from build123d import *

# Parameters (mm, degrees)
SKETCH1_W           = 1500
SKETCH1_H           = 1250
BOSS_EXTRUDE1_DEPTH = 150
CUT_EXTRUDE1_REACH  = 1633.908
LPATTERN1_COUNT     = 4
LPATTERN1_PITCH     = 150
LPATTERN1_COL_COUNT = 4
LPATTERN1_COL_PITCH = 150
CUT_EXTRUDE2_REACH  = 1467.435
SKETCH3_W           = 22
SKETCH3_H           = 11
LPATTERN2_COUNT     = 2
LPATTERN2_PITCH     = 525
LPATTERN2_COL_COUNT = 2
LPATTERN2_COL_PITCH = 525
CHAMFER1_SIZE       = 125


with BuildPart() as part:
    # Sketch1 → Boss-Extrude1 (new body)
    with BuildSketch(Plane(origin=(0, 0, 0), x_dir=(1, 0, 0), z_dir=(0, 1, 0))):
        Rectangle(SKETCH1_W, SKETCH1_H)
    extrude(amount=-BOSS_EXTRUDE1_DEPTH)

    # Sketch2 → Cut-Extrude1 (cut, up to next)
    with BuildSketch(Plane(origin=(750, 0, 0), x_dir=(0, 0, -1), z_dir=(1, 0, 0)), mode=Mode.PRIVATE) as cut_extrude1_sk1:
        Polygon((-11, 0), (11, 0), (11, -24), (18.5, -24), (18.5, -38), (-18.5, -38), (-18.5, -24), (-11, -24), align=None)
    cut_extrude1_tool1 = extrude(cut_extrude1_sk1.sketch, amount=-CUT_EXTRUDE1_REACH, mode=Mode.PRIVATE) & part.part
    cut_extrude1 = cut_extrude1_tool1.solids().sort_by_distance((750, -21.409178, 0))[0]
    add(cut_extrude1, mode=Mode.SUBTRACT)

    # LPattern1: Cut-Extrude1 ×4
    with Locations(*[(0, 0, -i * LPATTERN1_PITCH) for i in range(1, LPATTERN1_COUNT)]):
        add(cut_extrude1, mode=Mode.SUBTRACT)

    # LPattern1 col: Cut-Extrude1 ×4
    with Locations(*[(0, 0, i * LPATTERN1_COL_PITCH) for i in range(1, LPATTERN1_COL_COUNT)]):
        add(cut_extrude1, mode=Mode.SUBTRACT)

    # Cut-Extrude2: up to this face of the body (flat: up to its plane)
    cut_extrude2_end = Plane(part.part.faces().sort_by_distance((0, -75, 625))[0])
    # Sketch3 → Cut-Extrude2 (cut, up to the picked face)
    with BuildSketch(Plane(origin=(0, 0, -625), x_dir=(-1, 0, 0), z_dir=(0, 0, -1)), mode=Mode.PRIVATE) as cut_extrude2_sk1:
        with Locations((0, -5.5)):
            Rectangle(SKETCH3_W, SKETCH3_H)
    cut_extrude2_tool1 = split(extrude(cut_extrude2_sk1.sketch, amount=-CUT_EXTRUDE2_REACH, mode=Mode.PRIVATE), bisect_by=cut_extrude2_end, keep=Keep.BOTH, mode=Mode.PRIVATE)
    add(cut_extrude2_tool1.solids().sort_by(Axis((0, -5.5, -625), (0, 0, 1)))[0], mode=Mode.SUBTRACT)

    # LPattern2: Cut-Extrude1 ×2
    with Locations(*[(0, 0, -i * LPATTERN2_PITCH) for i in range(1, LPATTERN2_COUNT)]):
        add(cut_extrude1, mode=Mode.SUBTRACT)

    # LPattern2 col: Cut-Extrude1 ×2
    with Locations(*[(0, 0, i * LPATTERN2_COL_PITCH) for i in range(1, LPATTERN2_COL_COUNT)]):
        add(cut_extrude1, mode=Mode.SUBTRACT)

    # Chamfer1
    chamfer1_edges = [part.edges().sort_by_distance(p)[0] for p in [
        (-750, -75, 625),
        (-750, -75, -625),
        (750, -75, -625),
        (750, -75, 625),
    ]]
    chamfer(chamfer1_edges, length=CHAMFER1_SIZE)


solid = part.part
Geometry check sheet. Reference: the model listing, model coordinates, mm. A direction names the side the tool comes from. Coordinates: 2 decimals unless noted, no trailing zeros. Write each loop counter-clockwise with the first axis right and the second up, starting at its lowest first coordinate (ties: lowest second). Pieces come first, ordered by that corner, then holes. Notation, with made-up numbers: (67, 50.25) -> (100, 50.25) arc R16 cw to (100, 80.25) -> close; hole circle Ø11 at (39.5, 51). An arc over 180 degrees is marked (long way). One line per question, with ' | ' between items.
1. Cross-section at A-A on y = -88.5. Record the cut outline in (x, z), and give its area (3 significant figures).
Answers:
outline: (-750, -500) -> (-625, -625) -> (625, -625) -> (750, -500) -> (750, 500) -> (625, 625) -> (-625, 625) -> (-750, 500) -> close | area: 1,840,000 mm²
2. Thickness scan on probe 1 along Y at (x, z) = (127.5, 287); probe 2 along Z at (x, y) = (634, -59.5); probe 3 along Z at (x, y) = (668.5, -101). Record the ranges inside material, lowest first. Write a range as from..to.
Answers:
probe 1: y = -150..-38, -24..0 | probe 2: z = -616..616 | probe 3: z = -581.5..581.5
3. Depth check by flat-ended pin: pin 1 Ø17.5 at (x, z) = (-3.5, 219.5) entering from +Y; pin 2 Ø3.5 at (y, z) = (-3.5, -587) entering from +X; pin 3 Ø6.5 at (x, z) = (1.5, -595) entering from +Y; pin 4 Ø11 at (x, z) = (309, -528) entering from +Y. Enter the tip coordinate at first touch or a pass-through.
Answers:
pin 1: stops at y = 0 | pin 2: stops at x = 664.75 | pin 3: stops at y = -11 | pin 4: stops at y = -38
4. Draft check along Y on faces 3 (the flat face through (10, -38, 450)), 4 (the flat face through (375, 0, -376)), 5 (the flat face through (750, -74, 7)). Enter one of: +Y half, -Y half, draft (parallel to the pull), parting line (faces both ways), or undercut.
Answers:
face 3: undercut | face 4: +Y half | face 5: draft
5. Set-up check for faces 1 (the flat face through (10, -38, -150)), 2 (the flat face through (-9, -74, -625)): record each of +Z, -Z, +X, -X, +Y, -Y from which the full face is reachable in a straight line by a thin tool's end or side.
Answers:
face 1: +X, -X | face 2: -Z, +X, -X, +Y, -Y
